```python
from build123d import *

# Parameters (mm, degrees)
SKETCH1_R                                            = 19
SKETCH1_R_2                                          = 2.5
BOSS_EXTRUDE1_DEPTH                                  = 4
BOSS_EXTRUDE1_DEPTH_BACK                             = 4
CSK_FOR_ST2_2_CROSS_RECESSED_CTSK_HEAD_T_D           = 3
CSK_FOR_ST2_2_CROSS_RECESSED_CTSK_HEAD_T_DEPTH       = 10.1
CSK_FOR_ST2_2_CROSS_RECESSED_CTSK_HEAD_T_CSINK_D     = 4
CSK_FOR_ST2_2_CROSS_RECESSED_CTSK_HEAD_T_CSINK_ANGLE = 90
CSK_FOR_ST2_2_CROSS_RECESSED_CTSK_HEAD_T_TIP         = 0.901290929


with BuildPart() as part:
    # Sketch1 → Boss-Extrude1 (new body, two sides)
    with BuildSketch(Plane.XY) as boss_extrude1_sk:
        with BuildLine():
            ThreePointArc((-11.512732462, 25.318870955), (-19.705993339, 27.468960361), (-20.294700731, 19.018763212))
            ThreePointArc((-20.294700731, 19.018763212), (-19.374590067, 17.092564941), (-19.968337465, 15.042124148))
            ThreePointArc((-19.968337465, 15.042124148), (3e-08, -25), (19.968337429, 15.042124196))
            ThreePointArc((19.968337429, 15.042124196), (19.37459007, 17.09256497), (20.294700731, 19.018763212))
            ThreePointArc((20.294700731, 19.018763212), (19.705993339, 27.468960361), (11.512732462, 25.318870955))
            ThreePointArc((11.512732462, 25.318870955), (9.982940481, 23.830053075), (7.850361432, 23.735455028))
            ThreePointArc((7.850361432, 23.735455028), (4.5e-08, 25), (-7.850361347, 23.735455056))
            ThreePointArc((-7.850361347, 23.735455056), (-9.982940439, 23.830053057), (-11.512732462, 25.318870955))
        make_face()
        Circle(SKETCH1_R, mode=Mode.SUBTRACT)
        with Locations((-16.5, 23)):
            Circle(SKETCH1_R_2, mode=Mode.SUBTRACT)
        with Locations((16.5, 23)):
            Circle(SKETCH1_R_2, mode=Mode.SUBTRACT)
    extrude(amount=BOSS_EXTRUDE1_DEPTH)
    extrude(boss_extrude1_sk.sketch, amount=-BOSS_EXTRUDE1_DEPTH_BACK)

    # CSK for ST2.2 Cross recessed CTSK head t
    with Locations(Plane(origin=(0, 25, 0), x_dir=(1, 0, 0), z_dir=(0, 1, 0))):
        with Locations((0, 0)):
            CounterSinkHole(CSK_FOR_ST2_2_CROSS_RECESSED_CTSK_HEAD_T_D / 2, CSK_FOR_ST2_2_CROSS_RECESSED_CTSK_HEAD_T_CSINK_D / 2, depth=CSK_FOR_ST2_2_CROSS_RECESSED_CTSK_HEAD_T_DEPTH, counter_sink_angle=CSK_FOR_ST2_2_CROSS_RECESSED_CTSK_HEAD_T_CSINK_ANGLE)
            with Locations((0, 0, -(CSK_FOR_ST2_2_CROSS_RECESSED_CTSK_HEAD_T_DEPTH + CSK_FOR_ST2_2_CROSS_RECESSED_CTSK_HEAD_T_TIP / 2))):  # 118° drill point
                Cone(0, CSK_FOR_ST2_2_CROSS_RECESSED_CTSK_HEAD_T_D / 2, CSK_FOR_ST2_2_CROSS_RECESSED_CTSK_HEAD_T_TIP, mode=Mode.SUBTRACT)


solid = part.part
```
Can you work these out from the model? Positions are in its coordinate system, mm. Coordinates: 2 decimals unless noted, no trailing zeros. Loops run counter-clockwise (first coordinate to the right, second up) from the corner with the lowest first, then second, coordinate; pieces in that order, holes last. Notation, with made-up numbers: (-5.75, 43) -> (43.25, 43) arc R33 cw to (43.25, 74) -> close; hole circle Ø5 at (-33.75, 44). An arc over 180 degrees is marked (long way). Put each result on its own line as item: value. Start each with the question number.
Q1. Thinking about a two-plate mould opening in Z: for faces 1 (the face through (1.5, 21.68, -0.07)), 2 (the face through (-18, 25, 0)), 3 (the face through (0, 20, -4)), which applies, pulls with the +Z half, pulls with the -Z half, needs draft (parallel to the pull), parting line crosses it, or undercut?
Q2. I'm going to push flat-ended pins straight in: P1, Ø2, axis at x = 14.5, z = -1, coming from the -Y side; P2, Ø4, axis at x = -8.5, z = -1.5, coming from the -Y side. Where does each tip first touch, or does it pass through?
Q3. I want a section at C-C (y = -6). Write out the boundary of the cut face in (x, z).
Q4. If I drill on line 1 (Y direction, x = -16.5, z = -1.5); line 2 (Y direction, x = -16, z = -3.25); line 3 (Z direction, x = 0, y = 23.1), over which ranges is the centre line in solid material (lowest first)? Write a range as [from, to].
Q5. I want a section at A-A (x = 0). Write out the boundary of the cut face in (y, z), plus the area to 4 significant figures.
Q6. I want a section at B-B (y = 0). Write out the boundary of the cut face in (x, z).
Q7. I want a section at D-D (x = -16.5). Write out the boundary of the cut face in (y, z), plus the area to 3 significant figures.
Taken from the geometry:
1. face 1: undercut
1. face 2: needs draft
1. face 3: pulls with the -Z half
2. P1: stops at y = -21.04
2. P2: stops at y = -24.14
3. outline: (-24.27, -4) -> (-18.03, -4) -> (-18.03, 4) -> (-24.27, 4) -> close; (18.03, -4) -> (24.27, -4) -> (24.27, 4) -> (18.03, 4) -> close
4. line 1: y = [-18.78, -9.42], [9.42, 20.5], [25.5, 28.5]
4. line 2: y = [-19.21, -10.25], [10.25, 20.55], [25.45, 28.48]
4. line 3: z = [-4, -1.5], [1.5, 4]
5. outline: (-25, -4) -> (-19, -4) -> (-19, 4) -> (-25, 4) -> close; (19, -4) -> (25, -4) -> (25, -2) -> (24.5, -1.5) -> (19, -1.5) -> close; (19, 1.5) -> (24.5, 1.5) -> (25, 2) -> (25, 4) -> (19, 4) -> close
5. area: 77.75 mm2
6. outline: (-25, -4) -> (-19, -4) -> (-19, 4) -> (-25, 4) -> close; (19, -4) -> (25, -4) -> (25, 4) -> (19, 4) -> close
7. outline: (-18.78, -4) -> (-9.42, -4) -> (-9.42, 4) -> (-18.78, 4) -> close; (9.42, -4) -> (20.5, -4) -> (20.5, 4) -> (9.42, 4) -> close; (25.5, -4) -> (28.5, -4) -> (28.5, 4) -> (25.5, 4) -> close
7. area: 188 mm2
